Autodesk Inventor part; units mm, degrees
ref_plane "YZ Plane" through (0, 0, 0) normal (1, 0, 0) x (0, 1, 0)
ref_plane "XZ Plane" through (0, 0, 0) normal (0, 1, 0) x (-1, 0, 0)
ref_plane "XY Plane" through (0, 0, 0) normal (0, 0, 1) x (1, 0, 0)
sketch "Skizze1" plane through (0, 0, 0) normal (0, 0, 1) x (1, 0, 0)
  line L0 (-8.4, 0) -> (8.4, 0)
  line L1 (0, -2) -> (0, 12)
  line L2 (6, 10) -> (6, 0)
  line L3 (6, 0) -> (-6, 0)
  line L4 (-6, 0) -> (-6, 10)
  line L5 (4.5, 10) -> (4.5, 2)
  line L6 (4.5, 2) -> (-4.5, 2)
  line L7 (-4.5, 2) -> (-4.5, 10)
  line L8 (-6, 10) -> (-4.5, 10)
  line L9 (4.5, 10) -> (6, 10)
  point P0 (0, 0)
  dimension "d0" = 2
  dimension "d2" = 9
  dimension "d3" = 1.5
  dimension "d4" = 10
extrude "Extrusion1" add sketch "Skizze1" along normal blind 40
sketch "Skizze2" plane through (-6, 0, 0) normal (0, -1, 0) x (1, 0, 0)
  line L0 (0, 0) -> (12, 0)
  line L1 (12, 0) -> (12, 40)
  point P0 (6, 0)
  point P1 (6, 2.5)
  dimension "d7" = 2.5
  dimension "d8" = 6
hole "Bohrung1" at (0, 0, 2.5) direction (0, 1, 0) diameter 2.4 end through all countersink diameter 4.5 countersink angle 90
sketch "Skizze3" plane through (-6, 0, 0) normal (0, -1, 0) x (1, 0, 0)
  line L0 (0, 40) -> (12, 40)
  line L1 (0, 0) -> (0, 40)
  line L2 (3.5, 33.5) -> (3.5, 22.5)
  line L3 (8.5, 22.5) -> (8.5, 33.5)
  arc A0 (8.5, 33.5) -> (3.5, 33.5) centre (6, 33.5) ccw
  arc A1 (3.5, 22.5) -> (8.5, 22.5) centre (6, 22.5) ccw
  line L4 (0, 0) -> (12, 0)
  line L5 (6, 22.5) -> (6, 33.5)
  point P0 (6, 0)
  point P1 (6, 28)
  dimension "d36" = 4
  dimension "d37" = 20
  dimension "d38" = 6
  dimension "d39" = 5
extrude "Extrusion2" cut sketch "Skizze3" against normal through all
sketch "Skizze4" plane through (6, 0, 0) normal (1, 0, 0) x (0, 0, -1)
  line L0 (0, 10) -> (-40, 10)
  line L1 (-40, 0) -> (-40, 10)
  line L2 (0, 0) -> (-40, 0)
  line L3 (-35, 5) -> (-28, 5) construction
  line L4 (-35, 7.5) -> (-28, 7.5)
  line L5 (-28, 2.5) -> (-35, 2.5)
  arc A0 (-35, 7.5) -> (-35, 2.5) centre (-35, 5) ccw
  arc A1 (-28, 2.5) -> (-28, 7.5) centre (-28, 5) ccw
  circle A2 centre (-35, 5) radius 5
  point P0 (-31.5, 5)
  dimension "d25" = 5
  dimension "d26" = 7
  dimension "d27" = 5
  dimension "d28" = 5
  dimension "d35" = 7
extrude "Extrusion3" cut sketch "Skizze4" against normal through all contours A2 L5 A0 L4 | L4 A1 L5 A2 picked at (-33.3333, 5)
pattern_linear "Rechteckige Anordnung1" count 2 spacing 15 along (0, 0, -1) of "Extrusion3"
fillet "Rundung1" radius 5 2 edges at (-5.25, 10, 40) (5.25, 10, 40)
properties part number "13_1087_002" material "Kupfer"
Source: CAD feature listing. Evaluate the final solid. Frame: model axes, mm. A direction names the side the tool comes from. Round coordinates to 2 decimals unless told otherwise and drop trailing zeros. Write each loop counter-clockwise with the first axis right and the second up, starting at its lowest first coordinate (ties: lowest second). Pieces come first, ordered by that corner, then holes. Notation, with made-up numbers: (74.25, 68) - (126.25, 68) arc R16 cw to (126.25, 80) - close; hole circle Ø5 at (-31, 1). An arc over 180 degrees is marked (long way). Use CSV: the item, a comma, the result in double quotes. Start each with the question number.
(1) Mould query, pull axis Y, two halves, no side actions, for faces 1 (the face through (-5, 9, 38)), 2 (the face through (5.3, 4.9, 25.5)), 3 (the face through (-6, 2, 20)). Classes: pulls with the +Y half, pulls with the -Y half, needs draft (parallel to the pull), parting line crosses it, or undercut.
(2) Cut plane B-B, the plane z = 26.5. Return loops of the section in (x, y).
(3) Material intervals for probe 1 along Z at (x, y) = (0, 1.65); probe 2 along X at (y, z) = (8.75, 37); probe 3 along X at (y, z) = (0.5, 31), sorted ascending. Write a range as [from, to].
(4) First-contact query: pin 1 Ø1 at (x, z) = (-1.5, 6) entering from -Y; pin 2 Ø7 at (x, z) = (0.5, 12) entering from +Y. Flat tips, straight axial feed; report the tip coordinate or a pass-through.
(5) Set-up query: faces 4 (the face through (-5.2, 4.9, 25.5)), 5 (the face through (-0.1, 1.7, 0)), 6 (the face through (-4.5, 8, 20)), 7 (the face through (-2.5, 1, 28)). Return all of +Z, -Z, +X, -X, +Y, -Y with unobstructed straight access to the full face (end or side cutting, diameter ignored); none if empty.
(6) Cut plane C-C, the plane y = 5.5. Return loops of the section in (x, z).
(7) Cut plane A-A, the plane x = 5. Return loops of the section in (y, z), and give its area (3 significant figures).
(8) Cut plane D-D, the plane x = 0. Return loops of the section in (y, z).
Geometry says:
1,face 1,"pulls with the +Y half"
1,face 2,"undercut"
1,face 3,"needs draft"
2,outline,"(-6, 0) - (-2.5, 0) - (-2.5, 2) - (-4.5, 2) - (-4.5, 3) - (-6, 3) - close; (-6, 7) - (-4.5, 7) - (-4.5, 10) - (-6, 10) - close; (2.5, 0) - (6, 0) - (6, 3) - (4.5, 3) - (4.5, 2) - (2.5, 2) - close; (4.5, 7) - (6, 7) - (6, 10) - (4.5, 10) - close"
3,probe 1,"[0, 1.3], [3.7, 20], [36, 40]"
3,probe 2,"[-6, -4.5], [4.5, 6]"
3,probe 3,"[-6, -2.5], [2.5, 6]"
4,pin 1,"y = 0"
4,pin 2,"y = 2"
5,face 4,"+X, -X"
5,face 5,"-Z, +X, -X, +Y, -Y"
5,face 6,"+Z, -Z, +Y"
5,face 7,"+Y, -Y"
6,outline,"(-6, 0) - (-4.5, 0) - (-4.5, 10.55) - (-6, 10.55) - close; (-6, 22.45) - (-4.5, 22.45) - (-4.5, 25.55) - (-6, 25.55) - close; (-6, 37.45) - (-4.5, 37.45) - (-4.5, 39.97) - (-6, 39.97) - close; (4.5, 0) - (6, 0) - (6, 10.55) - (4.5, 10.55) - close; (4.5, 22.45) - (6, 22.45) - (6, 25.55) - (4.5, 25.55) - close; (4.5, 37.45) - (6, 37.45) - (6, 39.97) - (4.5, 39.97) - close"
7,outline,"(0, 0) - (10, 0) - (10, 35) arc R5 ccw to (5, 40) - (0, 40) - close; hole (2.5, 13) arc R2.5 ccw to (7.5, 13) - (7.5, 20) arc R2.5 ccw to (2.5, 20) - close; hole (2.5, 28) arc R2.5 ccw to (7.5, 28) - (7.5, 35) arc R2.5 ccw to (2.5, 35) - close"
7,area,"285 mm²"
8,outline,"(0, 0) - (2, 0) - (2, 1.3) - (1.05, 1.3) - (0, 0.25) - close; (0, 4.75) - (1.05, 3.7) - (2, 3.7) - (2, 20) - (0, 20) - close; (0, 36) - (2, 36) - (2, 40) - (0, 40) - close"
